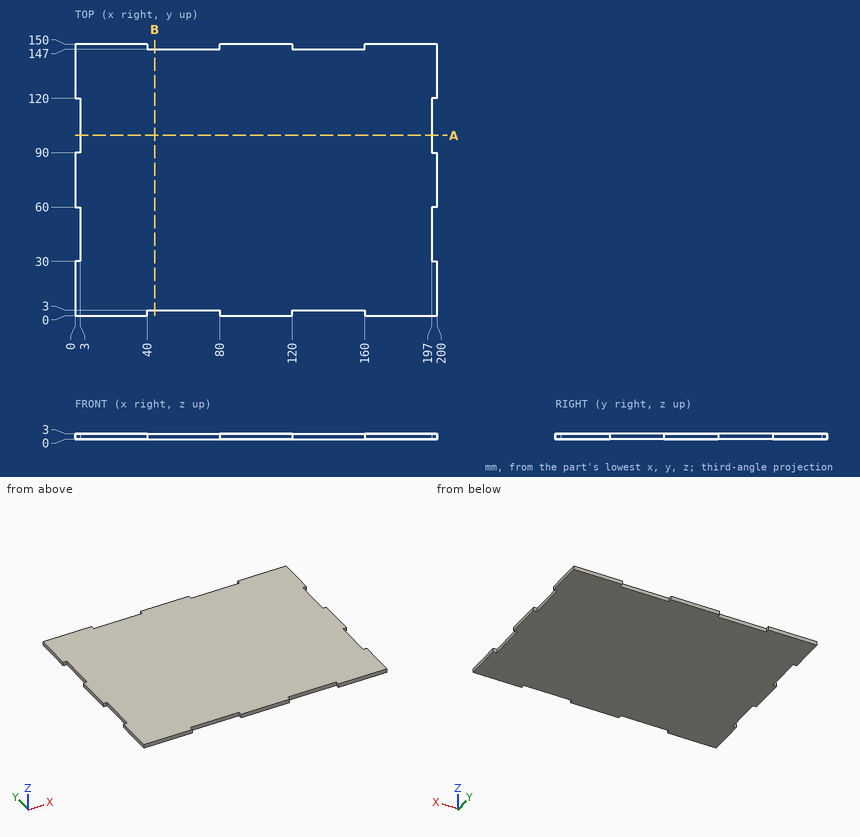
Input: dimensioned drawing with shaded views. Units: mm. Origin: part minimum x, y, z. Round coordinates to 2 decimals unless told otherwise and drop trailing zeros. Loops run counter-clockwise (first coordinate to the right, second up) from the corner with the lowest first, then second, coordinate; pieces in that order, holes last. Notation, with made-up numbers: (39.5, 7) -> (68.5, 7) arc R10 ccw to (68.5, 16) -> close; hole circle Ø9 at (-38, -7). An arc over 180 degrees is marked (long way). One line per item, written item: value.
(1) Material intervals for line 1 (X direction, y = 34, z = 2.75); line 2 (Y direction, x = 75, z = 1.3), sorted ascending. Write a range as [from, to].
Geometry check:
line 1: [3, 197]
line 2: [3, 147]
(2) Section B-B (x = 44). Return the cut outline in (y, z), plus the area to 3 significant figures.
Geometry check:
outline: (3, 0) -> (147, 0) -> (147, 3) -> (3, 3) -> close
area: 432 mm2
(3) Pin query (flat end, axial travel): pin 1 (1.5 mm diameter, centred on y = 105, z = 2, fed in from +X); pin 2 (1.5 mm diameter, centred on y = 108, z = 1, fed in from -X). Return the tip coordinate at first contact, or that it passes through.
Geometry check:
pin 1: x = 197
pin 2: x = 3
(4) Section A-A (y = 99.5). Return the cut outline in (x, z).
Geometry check:
outline: (3, 0) -> (197, 0) -> (197, 3) -> (3, 3) -> close
